from build123d import *

# Parameters (mm, degrees)
BOSS_EXTRUDE1_DEPTH     = 9.525
SKETCH2_R               = 3.16865
CUT_EXTRUDE1_DEPTH      = 45.650209115
CUT_EXTRUDE2_DEPTH      = 42.490532643
CUT_EXTRUDE2_DEPTH_BACK = 42.490532643
SKETCH3_R               = 5.55625


with BuildPart() as part:
    # Sketch1 → Boss-Extrude1 (new, symmetric)
    with BuildSketch(Plane.XY):
        with BuildLine():
            Line((7.5311, 39.243), (9.525, 39.243))
            Line((9.525, 39.243), (9.525, 10.16))
            Line((9.525, 10.16), (7.62, 10.16))
            ThreePointArc((7.62, 10.16), (0, 12.7), (-7.62, 10.16))
            Line((-7.62, 10.16), (-9.525, 10.16))
            Line((-9.525, 10.16), (-9.525, 39.243))
            Line((-9.525, 39.243), (-7.5311, 39.243))
            Line((-7.5311, 39.243), (-7.5311, 21.43125))
            ThreePointArc((-7.5311, 21.43125), (-5.671228061, 16.941121939), (-1.1811, 15.08125))
            Line((-1.1811, 15.08125), (1.1811, 15.08125))
            ThreePointArc((1.1811, 15.08125), (5.671228061, 16.941121939), (7.5311, 21.43125))
            Line((7.5311, 21.43125), (7.5311, 39.243))
        make_face()
    extrude(amount=BOSS_EXTRUDE1_DEPTH, both=True)

    # Sketch2 → Cut-Extrude1 (cut, through all)
    with BuildSketch(Plane(origin=(9.525, 0, 0), x_dir=(0, 0, -1), z_dir=(1, 0, 0))):
        with Locations(Location((0, 29.718, 0), (0, 0, 90))):
            Circle(SKETCH2_R)
        with BuildLine():
            Line((-9.525, 31.623), (-9.525, 39.243))
            Line((-9.525, 39.243), (-1.905, 39.243))
            ThreePointArc((-1.905, 39.243), (-7.293153673, 37.011153673), (-9.525, 31.623))
        make_face()
        with BuildLine():
            Line((9.525, 31.623), (9.525, 39.243))
            Line((9.525, 39.243), (1.905, 39.243))
            ThreePointArc((1.905, 39.243), (7.293153673, 37.011153673), (9.525, 31.623))
        make_face()
    extrude(amount=-CUT_EXTRUDE1_DEPTH, mode=Mode.SUBTRACT)

    # Sketch3 → Cut-Extrude2 (cut, two sides: drawn at the far end of the back side and taken through both)
    with BuildSketch(Plane(origin=(0, 0, 0), x_dir=(1, 0, 0), z_dir=(0, 1, 0)).offset(-CUT_EXTRUDE2_DEPTH_BACK)):
        with Locations(Location((0, 0, 0), (0, 0, 90))):
            Circle(SKETCH3_R)
    extrude(amount=CUT_EXTRUDE2_DEPTH + CUT_EXTRUDE2_DEPTH_BACK, mode=Mode.SUBTRACT)


solid = part.part
Build history of the part. All positions in model axes, mm. A direction names the side the tool comes from. Round coordinates to 2 decimals unless told otherwise and drop trailing zeros. Write each loop counter-clockwise with the first axis right and the second up, starting at its lowest first coordinate (ties: lowest second). Pieces come first, ordered by that corner, then holes. Notation, with made-up numbers: M 61.5,42 L 81.5,42 A10 cw 81.5,52 Z; hole C 38.5,61.25 d6. An arc over 180 degrees is marked long. Answer in a Markdown table with one row per item.
1. Flat gauge pins, fed straight in: P1, Ø2.5, axis at x = -0.5, z = -8.5, coming from the +Y side; P2, Ø4, axis at y = 29.718, z = 0, coming from the +X side; P3, Ø2, axis at x = -4.5, z = -4.5, coming from the -Y side; P4, Ø10, axis at x = -1.5, z = -1, coming from the -Y side. Where does each tip first touch, or does it go through?
Geometry check:
| item | result |
|---|---|
| P1 | y = 15.11 |
| P2 | through |
| P3 | y = 11.45 |
| P4 | y = 10.91 |
2. Which spindle directions (+Z, -Z, +X, -X, +Y, -Y) get a long thin tool onto all of the face, cutting with end or side? Do faces 4 (the face through (-6.422, 17.846, 0.133)), 5 (the face through (-8.514, 32.645, -1.214)). Say none if no direction does.
Geometry check:
| item | result |
|---|---|
| face 4 | +Z, -Z, +Y |
| face 5 | +X, -X |
3. Saw through at A-A (y = 23). List the corners of the cut face in (x, z) (3 decimals).
Geometry check:
| item | result |
|---|---|
| outline | M -9.525,-9.525 L -7.531,-9.525 L -7.531,9.525 L -9.525,9.525 Z; M 7.531,-9.525 L 9.525,-9.525 L 9.525,9.525 L 7.531,9.525 Z |
4. Mould opens along X. For faces 1 (the face through (9.525, 25, 0)), 2 (the face through (9, 10.16, 0)), 3 (the face through (0, 15.081, 8)) say: +X half, -X half, draft (parallel to the pull), parting line (faces both ways), or undercut.
Geometry check:
| item | result |
|---|---|
| face 1 | +X half |
| face 2 | draft |
| face 3 | undercut |
5. Saw through at C-C (x = 0). List the corners of the cut face in (y, z) (3 decimals).
Geometry check:
| item | result |
|---|---|
| outline | M 12.7,-9.525 L 15.081,-9.525 L 15.081,-5.556 L 12.7,-5.556 Z; M 12.7,5.556 L 15.081,5.556 L 15.081,9.525 L 12.7,9.525 Z |
6. Saw through at B-B (z = 0). List the corners of the cut face in (x, y) (3 decimals), and give its area (3 significant figures).
Geometry check:
| item | result |
|---|---|
| outline | M -9.525,10.16 L -7.62,10.16 A12.7 cw -5.556,11.42 L -5.556,16.829 A6.35 cw -7.531,21.431 L -7.531,26.549 L -9.525,26.549 Z; M -9.525,32.887 L -7.531,32.887 L -7.531,39.243 L -9.525,39.243 Z; M 5.556,11.42 A12.7 cw 7.62,10.16 L 9.525,10.16 L 9.525,26.549 L 7.531,26.549 L 7.531,21.431 A6.35 cw 5.556,16.829 Z; M 7.531,32.887 L 9.525,32.887 L 9.525,39.243 L 7.531,39.243 Z |
| area | 120 mm2 |
7. Probe L1, parallel to X at y = 14.25, z = 0 (3 decimals); L2, parallel to X at y = 34, z = -6.5 (3 decimals); L3, parallel to Y at x = 0.25, z = -8. List the from-to ranges inside material, lowest first. Write a range as [from, to].
Geometry check:
| item | result |
|---|---|
| L1 | [-9.525, -5.556], [5.556, 9.525] |
| L2 | [-9.525, -7.531], [7.531, 9.525] |
| L3 | [12.7, 15.08] |
8. Saw through at D-D (y = 13.5). List the corners of the cut face in (x, z) (1 decimal), and give its area (3 significant figures).
Geometry check:
| item | result |
|---|---|
| outline | M -9.5,-9.5 L 9.5,-9.5 L 9.5,9.5 L -9.5,9.5 Z; hole C 0,0 d11.1 |
| area | 266 mm2 |
